```python
from build123d import *

# Parameters (mm, degrees)
PAD_DEPTH         = 20
POCKET_DEPTH      = 6.001
POCKET_DEPTH_BACK = -31.001


with BuildPart() as part:
    # AdditivePipe: sweep along a path in Sketch
    with BuildLine(Plane.XY) as additivepipe_path:
        Line((0, 0), (0, 47))
    # Sketch001 → AdditivePipe (sweep)
    with BuildSketch(Plane.XZ):
        Polygon((-20, 6), (-20, -6), (-16, -6), (-9, -6), (9, -6), (16, -6), (20, -6), (20, 6), (16, 6), (16, 3), (9, 3), (-9, 3), (-16, 3), (-16, 6), align=None)
    sweep(path=additivepipe_path.line)

    # Sketch002 → Pad (new body, symmetric)
    with BuildSketch(Plane.YZ):
        Polygon((47, 6), (47, 17), (34, 31), (22, 31), (22, 17), (29, 17), (29, 3), (47, 3), align=None)
    extrude(amount=PAD_DEPTH, both=True)

    # Sketch003 → Pocket (cut, two sides)
    with BuildSketch(Plane.XY) as pocket_sk:
        with BuildLine():
            Line((-4.5, 0), (4.5, 0))
            Line((4.5, 0), (4.5, 7))
            ThreePointArc((4.5, 7), (0, 19.361903), (-4.5, 7))
            Line((-4.5, 0), (-4.5, 7))
        make_face()
    extrude(amount=-POCKET_DEPTH, mode=Mode.SUBTRACT)
    extrude(pocket_sk.sketch, amount=-POCKET_DEPTH_BACK, mode=Mode.SUBTRACT)


solid = part.part
```
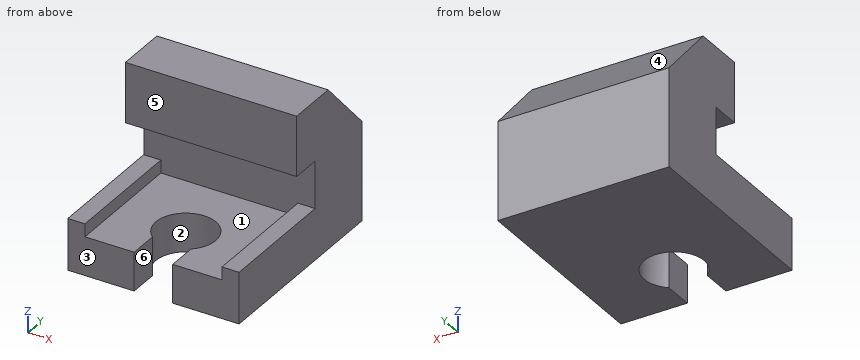
Input: part model. Units: mm. Frame: model coordinates. Face numbers are marked on the shaded views. A direction names the side the tool comes from. Round coordinates to 2 decimals unless told otherwise and drop trailing zeros. Loops run counter-clockwise (first coordinate to the right, second up) from the corner with the lowest first, then second, coordinate; pieces in that order, holes last. Notation, with made-up numbers: M 11.5,-6 L 45.5,-6 A23 ccw 45.5,33 Z; hole C 82.25,19.5 d3. An arc over 180 degrees is marked long. Answer in a Markdown table with one row per item. Add a question column.
1. Section C-C (y = 25.5). Output: boundary loops of the cut face in (x, z).
2. Ray query, probe 1 along Z at (x, y) = (-13.5, 23); probe 2 along Y at (x, z) = (17, 9); probe 3 along Z at (x, y) = (-17, 5). Return the intervals inside material, ascending.
3. Section B-B (x = -12). Output: boundary loops of the cut face in (y, z).
4. Section A-A (y = 5). Output: boundary loops of the cut face in (x, z), and give its area (3 significant figures).
5. Contact query for flat-ended pins moving along their axis: pin 1 (18 mm diameter, centred on x = 0, y = 12.36, fed in from +Z); pin 2 (8 mm diameter, centred on x = 3, z = 26.5, fed in from -Y); pin 3 (8 mm diameter, centred on y = 9.5, z = 11, fed in from +X); pin 4 (1.2 mm diameter, centred on x = -18, y = 18.5, fed in from +Z). Output: stop coordinate, or through.
6. Set-up query: the marked faces 4, 5 and 6. Return all of +Z, -Z, +X, -X, +Y, -Y with unobstructed straight access to the full face (end or side cutting, diameter ignored); none if empty.
7. Mould query, pull axis Y, two halves, no side actions, for the marked faces 1, 2 and 3. Classes: released by +Y, released by -Y, zero draft, split by the parting line, or undercut.
8. Section D-D (z = 11.5). Output: boundary loops of the cut face in (x, y), and give its area (3 significant figures).
Values follow:
| question | item | result |
|---|---|---|
| 1 | outline | M -20,-6 L 20,-6 L 20,6 L 16,6 L 16,3 L -16,3 L -16,6 L -20,6 Z; M -20,17 L 20,17 L 20,31 L -20,31 Z |
| 2 | probe 1 | -6 to 3, 17 to 31 |
| 2 | probe 2 | 29 to 47 |
| 2 | probe 3 | -6 to 6 |
| 3 | outline | M 0,-6 L 47,-6 L 47,17 L 34,31 L 22,31 L 22,17 L 29,17 L 29,3 L 0,3 Z |
| 4 | outline | M -20,-6 L -4.5,-6 L -4.5,3 L -16,3 L -16,6 L -20,6 Z; M 4.5,-6 L 20,-6 L 20,6 L 16,6 L 16,3 L 4.5,3 Z |
| 4 | area | 303 mm^2 |
| 5 | pin 1 | z = 3 |
| 5 | pin 2 | y = 22 |
| 5 | pin 3 | through |
| 5 | pin 4 | z = 6 |
| 6 | face 4 | +Z, +X, -X, +Y |
| 6 | face 5 | +Z, +X, -X, -Y |
| 6 | face 6 | +Z, -Z, -Y |
| 7 | face 1 | zero draft |
| 7 | face 2 | undercut |
| 7 | face 3 | released by -Y |
| 8 | outline | M -20,29 L 20,29 L 20,47 L -20,47 Z |
| 8 | area | 720 mm^2 |
